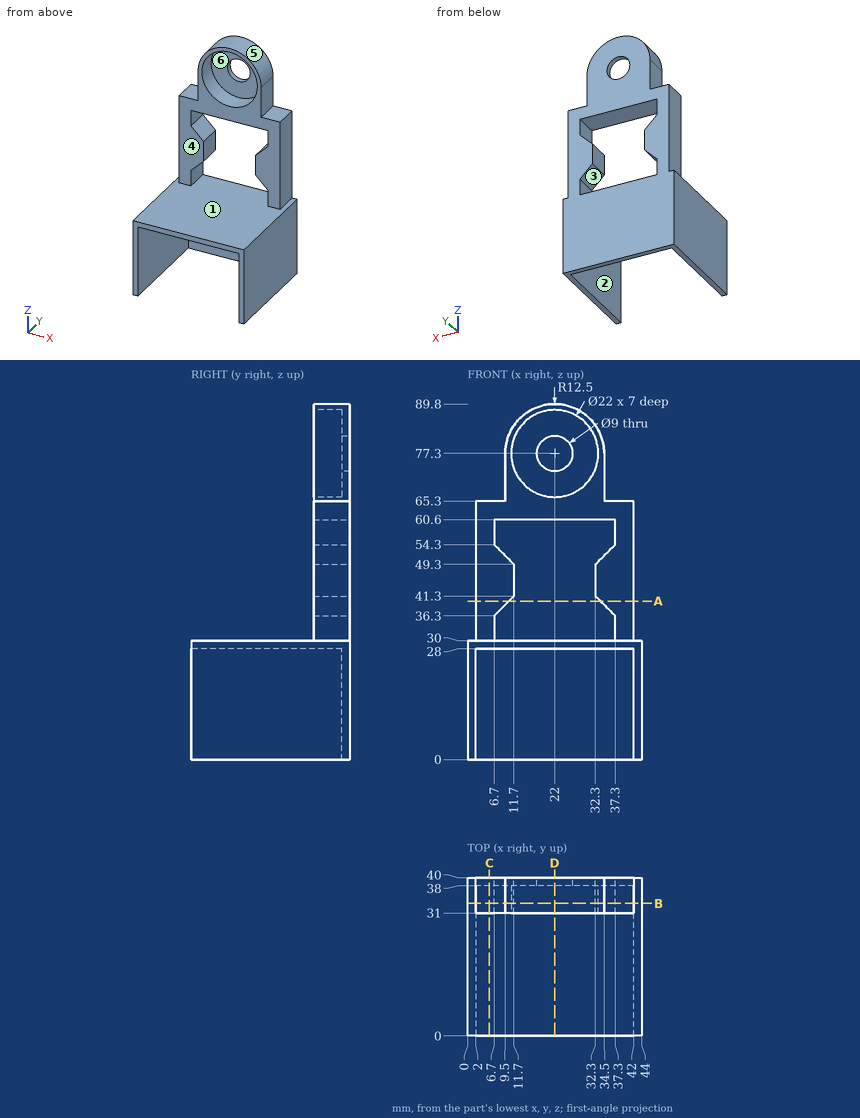
Could you check a few things on this drawing? It's one solid part, dimensions in mm from its lowest x, y, z. A direction names the side the tool comes from. Give positions to 0.01 mm unless a question says otherwise; leave off trailing zeros. Order: outer loops, then holes, each group sorted by start corner. A loop starts at its lowest first (then second) coordinate and runs counter-clockwise, first axis right, second up. Notation, with made-up numbers: (30, 8.25) - (52, 8.25) arc R24 ccw to (52, 37.25) - close; hole circle Ø2 at (15, -2.75). An arc over 180 degrees is marked (long way). Return JSON: item names as keys, results as strings. Group by question number.
Q1. Suppose I cut it at A-A, the plane z = 40. Please give me the cut outline in (x, y), and give its area (3 significant figures).
Q2. Which directions (+Z, -Z, +X, -X, +Y, -Y) give clear straight access to the entire face, cutting with the end or side of a thin tool? Please do the marked faces 1, 2 and 3.
Q3. Suppose I cut it at C-C, the plane x = 5.5. Please give me the cut outline in (y, z), and give its area (3 significant figures).
Q4. Thinking about a two-plate mould opening in X: for the marked faces 4, 5 and 6, which applies, pulls with the +X half, pulls with the -X half, needs draft (parallel to the pull), parting line crosses it, or undercut?
Q5. Suppose I cut it at B-B, the plane y = 33.5. State how many separate pieces and enclosed holes the cut face has, and give its area (3 significant figures).
Q6. Please list where these lines run through material, in increasing order: line 1 along Z through (x, y) = (22, 33); line 2 along X through (y, z) = (38, 47.5); line 3 along X through (y, z) = (39, 77). Write a range as [from, to].
Q7. Will these pins go through, and if not, where does the flat tip stop? pin 1 Ø17.5 at (x, z) = (22, 72.5) entering from -Y; pin 2 Ø2.5 at (y, z) = (37, 44) entering from +X; pin 3 Ø1 at (x, y) = (27.5, 11) entering from +Z; pin 4 Ø1 at (y, z) = (29, 46) entering from +X.
Q8. Suppose I cut it at D-D, the plane x = 22. Please give me the cut outline in (y, z).
Resolved:
{
 "1": {"outline": "(2, 31) - (10.4, 31) - (10.4, 40) - (2, 40) - close; (33.6, 31) - (42, 31) - (42, 40) - (33.6, 40) - close", "area": "151 mm2"},
 "2": {"face 1": "-Y", "face 2": "-Z, -Y", "face 3": "+Y, -Y"},
 "3": {"outline": "(0, 28) - (38, 28) - (38, 0) - (40, 0) - (40, 65.3) - (31, 65.3) - (31, 30) - (0, 30) - close", "area": "454 mm2"},
 "4": {"face 4": "needs draft", "face 5": "parting line crosses it", "face 6": "undercut"},
 "5": {"separate pieces": "1", "enclosed holes": "2", "area": "971 mm2"},
 "6": {"line 1": "z = [28, 30], [60.6, 66.3], [88.3, 89.8]", "line 2": "x = [2, 11.7], [32.3, 42]", "line 3": "x = [9.5, 17.51], [26.49, 34.5]"},
 "7": {"pin 1": "stops at y = 31", "pin 2": "stops at x = 42", "pin 3": "stops at z = 30", "pin 4": "passes through"},
 "8": {"outline": "(0, 28) - (38, 28) - (38, 0) - (40, 0) - (40, 30) - (0, 30) - close; (31, 60.6) - (40, 60.6) - (40, 72.8) - (38, 72.8) - (38, 66.3) - (31, 66.3) - close; (31, 88.3) - (38, 88.3) - (38, 81.8) - (40, 81.8) - (40, 89.8) - (31, 89.8) - close"}
}
